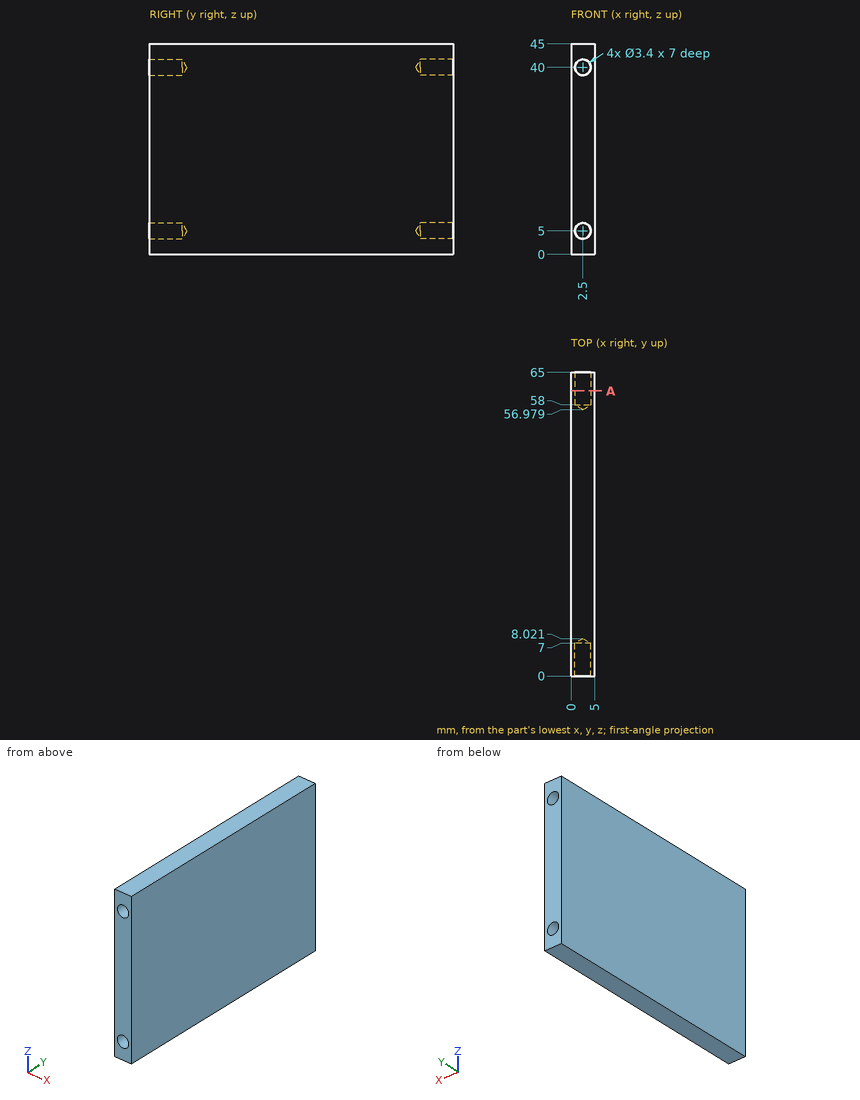
Part print with two shaded views. Sizes in mm from the minimum x, y, z corner. Coordinates: 2 decimals unless noted, no trailing zeros. Write each loop counter-clockwise with the first axis right and the second up, starting at its lowest first coordinate (ties: lowest second). Pieces come first, ordered by that corner, then holes. Notation, with made-up numbers: M 24.25,75 L 60.25,75 A22 ccw 60.25,92 Z; hole C 87.5,23 d3. An arc over 180 degrees is marked long. Return JSON: item names as keys, results as strings.
Item 1: Drop flat-ended pins along their axis: pin 1 Ø1 at (x, z) = (4, 37.5) entering from -Y; pin 2 Ø2.5 at (x, z) = (2.5, 40) entering from +Y; pin 3 Ø2.5 at (x, z) = (2.5, 5) entering from -Y; pin 4 Ø3 at (x, z) = (2.5, 40) entering from -Y. Give the stop position or say it passes through.
Findings below:
{"pin 1": "stops at y = 0", "pin 2": "stops at y = 57.73", "pin 3": "stops at y = 7.27", "pin 4": "stops at y = 7.12"}
Item 2: Slice it at A-A, the plane y = 61. Write the cut outline in (x, z), and give its area (3 significant figures).
Findings below:
{"outline": "M 0,0 L 5,0 L 5,45 L 0,45 Z; hole C 2.5,5 d3.4; hole C 2.5,40 d3.4", "area": "207 mm2"}
Item 3: Probe line 1 (Z direction, x = 2.6, y = 60.5); line 2 (X direction, y = 62.5, z = 5). List the from-to ranges inside material, lowest first. Write a range as from..to.
Findings below:
{"line 1": "z = 0..3.3, 6.7..38.3, 41.7..45", "line 2": "x = 0..0.8, 4.2..5"}
